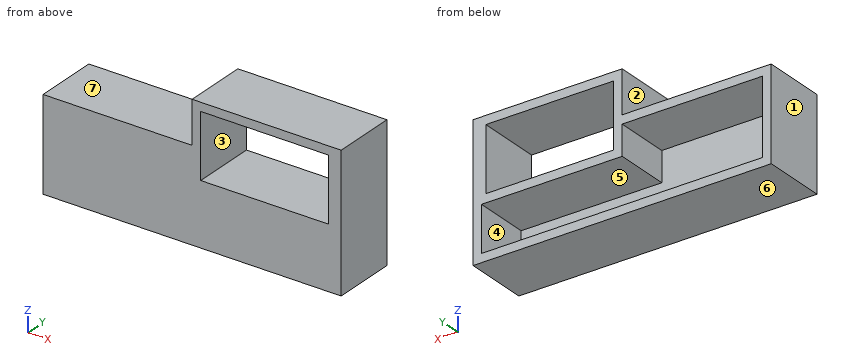
```python
from build123d import *

# Parameters (mm, degrees)
F1_DEPTH = 457.2
F2_W     = 914.4
F2_H     = 457.2
F3_DEPTH = 457.2
F4_T     = -60.96


# Not quite as in the source:
# - a shell that OpenCascade refuses in one call is made with other operations: the cavity is built on its own and cut out


with BuildPart() as f1:
    # F0 (on Front) → F1 (new body)
    with BuildSketch(Plane.XZ):
        Polygon((-0.0530799283, 304.7990856), (-0.0530799283, 0), (-1066.8530799283, 0), (-1066.8530799283, -660.401016), (-0.0530799283, -660.401016), (1066.7469200717, -660.401016), (1066.7469200717, 304.7990856), align=None)
    extrude(amount=-F1_DEPTH)

    # F2 (on face) → F3 (cut, through all)
    with BuildSketch(Plane.XZ):
        with Locations((518.1069200717, 15.2390856)):
            Rectangle(F2_W, F2_H)
    extrude(amount=-F3_DEPTH, mode=Mode.SUBTRACT)

    # F4: a shell. OpenCascade refuses it in one call, so the cavity is built on its own and cut out:
    # the body offset inwards by the wall thickness, plus a prism from it out through each open face.
    f4_core = offset(f1.part, amount=F4_T, kind=Kind.INTERSECTION, mode=Mode.PRIVATE)
    f4_exits = [f4_core.faces().sort_by_distance(p)[0] for p in [
        (-124.304275, 396.24, -370.362523),
    ]]
    add(f4_core, mode=Mode.SUBTRACT)
    extrude(f4_exits, amount=-F4_T, mode=Mode.SUBTRACT)


solid = f1.part
```
The listing builds one solid part. Answer for the finished solid, in the listing's coordinates (mm). Face numbers are marked on the shaded views. A direction names the side the tool comes from. Give positions to 0.01 mm unless a question says otherwise; leave off trailing zeros. Order: outer loops, then holes, each group sorted by start corner. A loop starts at its lowest first (then second) coordinate and runs counter-clockwise, first axis right, second up. Notation, with made-up numbers: (48.5, -30.5) -> (77.5, -30.5) arc R11 ccw to (77.5, -22.5) -> close; hole circle Ø4 at (81, 26). An arc over 180 degrees is marked (long way). Answer as a JSON object with one key per item and string values. Group by question number.
Item 1: The part is cut by section C-C on x = 637.5. Write down the section's boundary in (y, z).
Item 2: Determine the mould class of the marked faces 5, 6 and 7 for opening direction Z: pulls with the +Z half, pulls with the -Z half, needs draft (parallel to the pull), parting line crosses it, or undercut.
Item 3: The part is cut by section A-A on z = 141. Write down the section's boundary in (x, y).
Item 4: The part is cut by section B-B on y = 153.5. Write down the section's boundary in (x, z), and give its area (3 significant figures).
Item 5: Consider L1, parallel to X at y = 149, z = -146.5; L2, parallel to Z at x = 658.5, y = 310; L3, parallel to X at y = 332, z = 195. Determine where each line is inside the solid, lowest interval first. Write a range as from..to.
Item 6: The part is cut by section D-D on y = 33. Write down the section's boundary in (x, z), and give its area (3 significant figures).
Item 7: Flat-ended cylindrical pins translate along their axes: pin 1 (12 mm diameter, centred on x = 614.5, z = -346.5, fed in from -Y); pin 2 (10 mm diameter, centred on y = 155, z = 29, fed in from -X). Find the tip coordinate at first contact, or state that the pin passes through.
Item 8: A tool of negligible diameter and unlimited length cuts with its end or side. For the marked faces 1, 2, 3 and 4, from which of +Z, -Z, +X, -X, +Y, -Y can it reach the whole face along a straight path? Write none if from no direction.
Result set:
{
 "1": {"outline": "(0, -660.4) -> (457.2, -660.4) -> (457.2, -599.44) -> (60.96, -599.44) -> (60.96, -274.32) -> (457.2, -274.32) -> (457.2, -213.36) -> (0, -213.36) -> close; (0, 243.84) -> (457.2, 243.84) -> (457.2, 304.8) -> (0, 304.8) -> close"},
 "2": {"face 5": "undercut", "face 6": "pulls with the -Z half", "face 7": "pulls with the +Z half"},
 "3": {"outline": "(-0.05, 0) -> (60.91, 0) -> (60.91, 457.2) -> (-0.05, 457.2) -> close; (975.31, 0) -> (1066.75, 0) -> (1066.75, 457.2) -> (975.31, 457.2) -> close"},
 "4": {"outline": "(-1066.85, -660.4) -> (1066.75, -660.4) -> (1066.75, 304.8) -> (-0.05, 304.8) -> (-0.05, 0) -> (-1066.85, 0) -> close; hole (-1005.89, -599.44) -> (1005.79, -599.44) -> (1005.79, -274.32) -> (-0.05, -274.32) -> (-0.05, -60.96) -> (-1005.89, -60.96) -> close; hole (60.91, -213.36) -> (975.31, -213.36) -> (975.31, 243.84) -> (60.91, 243.84) -> close", "area": "447,000 mm²"},
 "5": {"L1": "-1066.85..-1005.89, -0.05..60.91, 975.31..1066.75", "L2": "-660.4..-599.44, -274.32..-213.36, 243.84..304.8", "L3": "-0.05..60.91, 975.31..1066.75"},
 "6": {"outline": "(-1066.85, -660.4) -> (1066.75, -660.4) -> (1066.75, 304.8) -> (-0.05, 304.8) -> (-0.05, 0) -> (-1066.85, 0) -> close; hole (60.91, -213.36) -> (975.31, -213.36) -> (975.31, 243.84) -> (60.91, 243.84) -> close", "area": "1,320,000 mm²"},
 "7": {"pin 1": "y = 0", "pin 2": "x = -0.05"},
 "8": {"face 1": "+Z, -Z, -X, +Y, -Y", "face 2": "+Z, -X, +Y, -Y", "face 3": "+Y, -Y", "face 4": "+Y"}
}
